Can you work these out from the model? Positions are in its coordinate system, mm. Face numbers are marked on the shaded views. A direction names the side the tool comes from. Coordinates: 2 decimals unless noted, no trailing zeros. Order: outer loops, then holes, each group sorted by start corner. A loop starts at its lowest first (then second) coordinate and runs counter-clockwise, first axis right, second up. Notation, with made-up numbers: (-20.75, 15.25) - (-15.75, 15.25) arc R17 ccw to (-15.75, 30.25) - close; hole circle Ø7 at (14, -31.75). An arc over 180 degrees is marked (long way). Return JSON: item names as keys, results as strings. Group by question number.
1) Imagine slicing it at C-C (x = -20.5). Write out the boundary of the cut face in (y, z), and give its area (3 significant figures).
2) Imagine slicing it at A-A (z = 0). Write out the boundary of the cut face in (x, y).
3) Imagine slicing it at B-B (y = -5). Write out the boundary of the cut face in (x, z).
4) If we mould it in two halves opening along X, with no side actions, what happens to the marked faces 1 and 2? For each: pulls with the +X half, pulls with the -X half, needs draft (parallel to the pull), parting line crosses it, or undercut.
5) If I drill on line 1 along Y through (x, z) = (11.5, -2.75); line 2 along X through (y, z) = (-5.25, 1.5); line 3 along X through (y, z) = (-7.5, 1), over which ranges is the centre line in solid material (lowest first)?
6) Which directions (+Z, -Z, +X, -X, +Y, -Y) give clear straight access to the entire face, cutting with the end or side of a thin tool? Please do the marked faces 3 and 4.
7) For pin 1 Ø6 at (x, y) = (-19.5, -13) entering from -Z; pin 2 Ø4 at (y, z) = (-14.5, 1.5) entering from +X; pin 3 Ø1.5 at (x, z) = (16.5, -3.5) entering from -Y, each with a flat end and sliding along its axis, tell me the tip position at first contact or that it passes through.
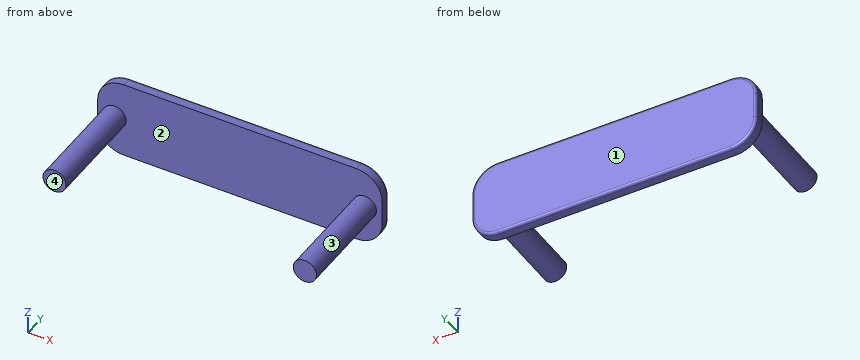
```python
from build123d import *

# Parameters (mm, degrees)
F1_DEPTH = 2
F2_R     = 0.5
F3_R     = 2.25
F4_DEPTH = 20


with BuildPart() as f1:
    # F0 (on Front) → F1 (new body)
    with BuildSketch(Plane.XZ):
        with BuildLine():
            Line((22.5, 7.5), (-22.5, 7.5))
            ThreePointArc((-22.5, 7.5), (-26.035534, 6.035534), (-27.5, 2.5))
            Line((-27.5, 2.5), (-27.5, -2.5))
            ThreePointArc((-27.5, -2.5), (-26.035534, -6.035534), (-22.5, -7.5))
            Line((-22.5, -7.5), (22.5, -7.5))
            ThreePointArc((22.5, -7.5), (26.035534, -6.035534), (27.5, -2.5))
            Line((27.5, -2.5), (27.5, 2.5))
            ThreePointArc((27.5, 2.5), (26.035534, 6.035534), (22.5, 7.5))
        make_face()
    extrude(amount=-F1_DEPTH)

    # F2
    f2_edges = [f1.edges().sort_by_distance(p)[0] for p in [
        (0, 2, 7.5),
        (-26.035534, 2, 6.035534),
        (-27.5, 2, 0),
        (-26.035534, 2, -6.035534),
        (0, 2, -7.5),
        (26.035534, 2, -6.035534),
        (27.5, 2, 0),
        (26.035534, 2, 6.035534),
    ]]
    fillet(f2_edges, radius=F2_R)

    # F3 (on face) → F4 (join)
    with BuildSketch(Plane.XZ):
        with Locations((24.155941, 0)):
            Circle(F3_R)
        with Locations((-24.244059, 0)):
            Circle(F3_R)
    extrude(amount=F4_DEPTH)


solid = f1.part
```
Calculated:
{
 "1": {"outline": "(0, -7.5) - (1.5, -7.5) arc R0.5 ccw to (2, -7) - (2, 7) arc R0.5 ccw to (1.5, 7.5) - (0, 7.5) - close", "area": "29.9 mm2"},
 "2": {"outline": "(-27.5, 0) - (-26.49, 0) - (-26.49, -20) - (-21.99, -20) - (-21.99, 0) - (21.91, 0) - (21.91, -20) - (26.41, -20) - (26.41, 0) - (27.5, 0) - (27.5, 1.5) arc R0.5 ccw to (27, 2) - (-27, 2) arc R0.5 ccw to (-27.5, 1.5) - close"},
 "3": {"outline": "circle Ø4.5 at (-24.24, 0); circle Ø4.5 at (24.16, 0)"},
 "4": {"face 1": "needs draft", "face 2": "undercut"},
 "5": {"line 1": "0 to 2", "line 2": "-25.92 to -22.57, 22.48 to 25.83", "line 3": "-26.26 to -22.23, 22.14 to 26.17"},
 "6": {"face 3": "-Y", "face 4": "+Z, -Z, +X, -X, -Y"},
 "7": {"pin 1": "z = -1.42", "pin 2": "x = 26.41", "pin 3": "y = 0"}
}
